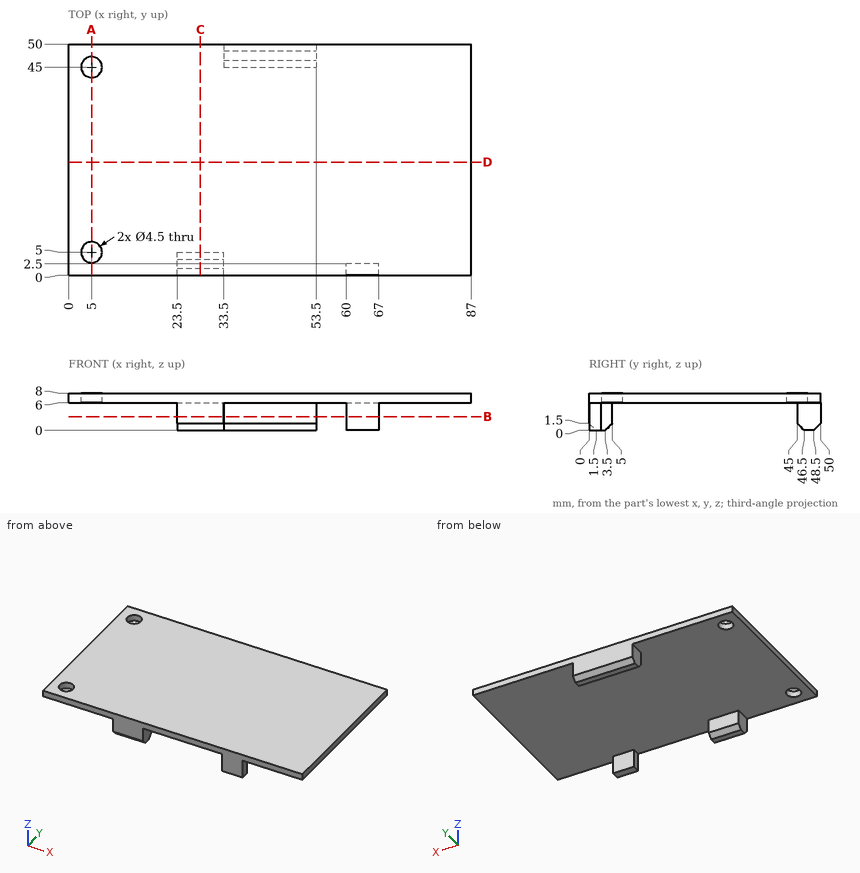
Can you work these out from the drawing? Everything is in mm from the part's minimum corner. Round coordinates to 2 decimals unless told otherwise and drop trailing zeros. Write each loop counter-clockwise with the first axis right and the second up, starting at its lowest first coordinate (ties: lowest second). Pieces come first, ordered by that corner, then holes.
1. Suppose I cut it at D-D (y = 24.5). List the corners of the cut face in (x, z) for me, and give its area (3 significant figures).
2. Will these pins go through, and if not, where does the flat tip stop? pin 1 Ø3.5 at (x, y) = (5, 5) entering from -Z; pin 2 Ø1.5 at (y, z) = (46.5, 3.5) entering from +X; pin 3 Ø8 at (x, y) = (35, 27.5) entering from -Z; pin 4 Ø2.5 at (y, z) = (48, 2) entering from -X.
3. Suppose I cut it at C-C (x = 28.5). List the corners of the cut face in (y, z) for me, and give its area (3 significant figures).
4. Suppose I cut it at A-A (x = 5). List the corners of the cut face in (y, z) for me.
5. I need wall thicknesses on L1, parallel to Y at x = 5, z = 7; L2, parallel to Y at x = 42.5, z = 4.5; L3, parallel to Z at x = 63, y = 36. Which ranges of each line are inside material? Lowest first, please.
6. Suppose I cut it at B-B (z = 3). List the corners of the cut face in (x, y) for me, and give its area (4 significant figures).
Answer sheet:
1. outline: (0, 6) - (87, 6) - (87, 8) - (0, 8) - close
1. area: 174 mm2
2. pin 1: passes through
2. pin 2: stops at x = 53.5
2. pin 3: stops at z = 6
2. pin 4: stops at x = 33.5
3. outline: (0, 1.5) - (1.5, 0) - (3.5, 0) - (5, 1.5) - (5, 6) - (50, 6) - (50, 8) - (0, 8) - close
3. area: 128 mm2
4. outline: (0, 6) - (2.75, 6) - (2.75, 8) - (0, 8) - close; (7.25, 6) - (42.75, 6) - (42.75, 8) - (7.25, 8) - close; (47.25, 6) - (50, 6) - (50, 8) - (47.25, 8) - close
5. L1: y = 0 to 2.75, 7.25 to 42.75, 47.25 to 50
5. L2: y = 45 to 50
5. L3: z = 6 to 8
6. outline: (23.5, 0) - (33.5, 0) - (33.5, 5) - (23.5, 5) - close; (33.5, 45) - (53.5, 45) - (53.5, 50) - (33.5, 50) - close; (60, 0) - (67, 0) - (67, 2.5) - (60, 2.5) - close
6. area: 167.5 mm2
